```python
from build123d import *

# Parameters (mm, degrees)
F0_R     = 3.175
F1_DEPTH = 152.4
F2_R     = 3.175
F3_DEPTH = 12.7


# Not quite as in the source:
# - a feature names something its author has since deleted; it is built from what else it names


with BuildPart() as f1:
    # F0 (on Right) → F1 (new body)
    with BuildSketch(Plane.YZ):
        with Locations((0, -3.175)):
            Circle(F0_R)
    extrude(amount=F1_DEPTH)

    # F2 (on Front) → F3 (join, symmetric)
    with BuildSketch(Plane.XZ):
        with BuildLine():
            ThreePointArc((92.075, 0), (88.9, 3.175), (85.725, 0))
            ThreePointArc((85.725, 0), (88.9, -3.175), (92.075, 0))
        make_face()
        with Locations((63.5, 0)):
            Circle(F2_R)
    extrude(amount=F3_DEPTH, both=True)


solid = f1.part
```
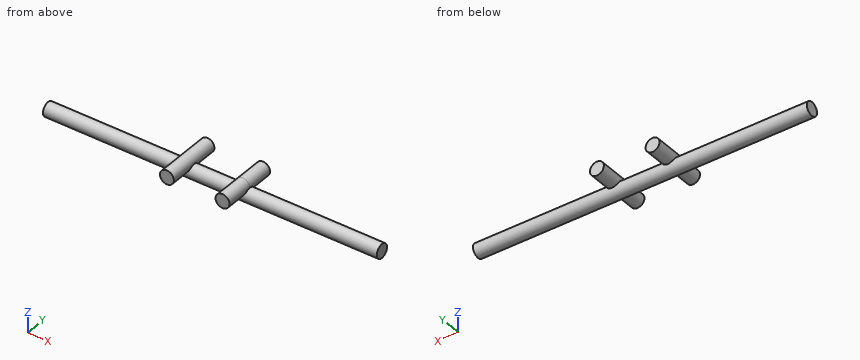
Geometry: final body of the model. Coordinates: model frame, mm. Round coordinates to 2 decimals unless told otherwise and drop trailing zeros. Order: outer loops, then holes, each group sorted by start corner. A loop starts at its lowest first (then second) coordinate and runs counter-clockwise, first axis right, second up. Notation, with made-up numbers: (24, 39.25) - (70, 39.25) arc R14 ccw to (70, 62.25) - close; hole circle Ø7 at (63.25, 15.25). An arc over 180 degrees is marked (long way). Use CSV: the item, a comma, the result in double quotes. Start each with the question number.
Q1. Section query B-B (x = 88.9). Return loops of the section in (y, z) (3 decimals), and give its area (3 significant figures).
Q2. Material intervals for line 1 along X through (y, z) = (7, -0.25); line 2 along Y through (x, z) = (56.5, -3.5); line 3 along X through (y, z) = (10.5, -1.75), sorted ascending. Write a range as from..to.
Q3. Section query D-D (x = 71.5). Return loops of the section in (y, z) (3 decimals), and give its area (3 significant figures).
Q4. Section query C-C (y = 6.5). Return loops of the section in (x, z) (3 decimals).
Q5. First-contact query: pin 1 (3 mm diameter, centred on x = 23, z = 0.5, fed in from -Y); pin 2 (1 mm diameter, centred on x = 58.5, y = -2, fed in from +Z); pin 3 (4 mm diameter, centred on x = 49, y = -3, fed in from +Z). Flat tips, straight axial feed; report the tip coordinate or a pass-through.
Q6. Section query A-A (z = 1.25). Return loops of the section in (x, y), and give its area (3 significant figures).
Result set:
1,outline,"(-12.7, -3.175) - (-3.175, -3.175) arc R3.175 ccw to (3.175, -3.175) - (12.7, -3.175) - (12.7, 3.175) - (-12.7, 3.175) - close"
1,area,"177 mm2"
2,line 1,"x = 60.33..66.67, 85.73..92.07"
2,line 2,"y = -3.16..3.16"
2,line 3,"x = 60.85..66.15, 86.25..91.55"
3,outline,"circle Ø6.35 at (0, -3.175)"
3,area,"31.7 mm2"
4,outline,"circle Ø6.35 at (63.5, 0); circle Ø6.35 at (88.9, 0)"
5,pin 1,"stops at y = -2.31"
5,pin 2,"stops at z = -0.38"
5,pin 3,"stops at z = -0.16"
6,outline,"(60.58, -12.7) - (66.42, -12.7) - (66.42, 12.7) - (60.58, 12.7) - close; (85.98, -12.7) - (91.82, -12.7) - (91.82, 12.7) - (85.98, 12.7) - close"
6,area,"297 mm2"
